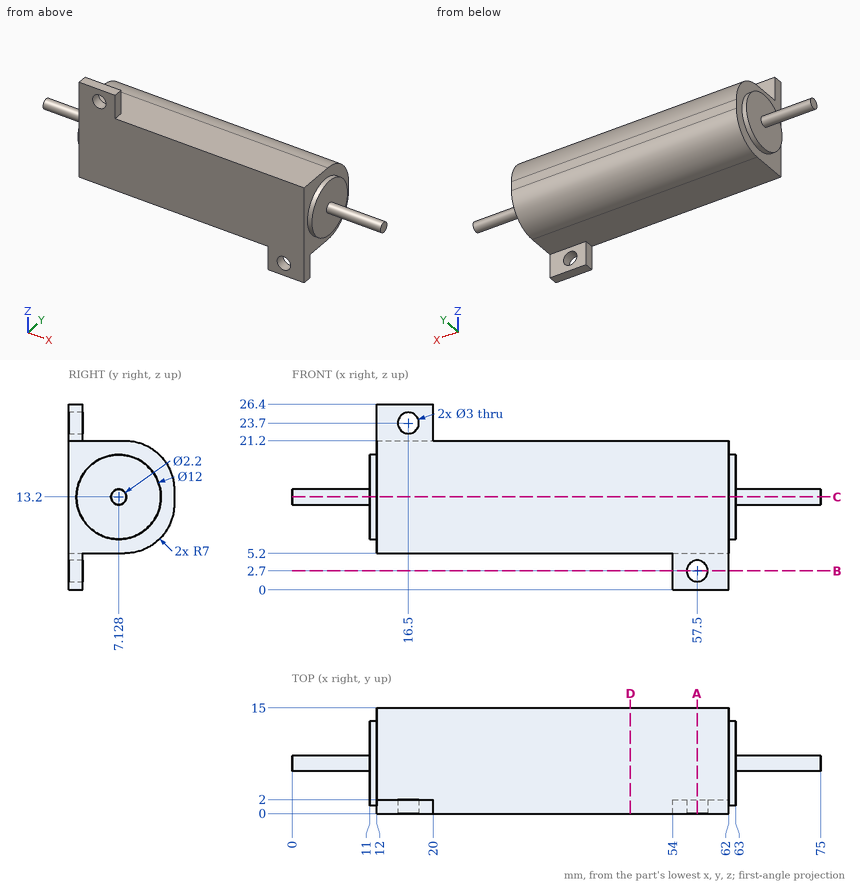
Design review of the part shown in the three views and the two pictorial views. Dimensions are in mm from the part's minimum x, y and z. Round coordinates to 2 decimals unless told otherwise and drop trailing zeros. Loops run counter-clockwise (first coordinate to the right, second up) from the corner with the lowest first, then second, coordinate; pieces in that order, holes last. Notation, with made-up numbers: M -18,57 L 40,57 A18 ccw 40,76 Z; hole C 74.5,49.5 d4. An arc over 180 degrees is marked long. Answer as a JSON object with one key per item and string values.
Item 1: Clearance check with flat-ended pins moving along their axes: P1, Ø1, axis at y = 1.5, z = 25, coming from the +X side; P2, Ø1.5, axis at x = 47.5, y = 12.5, coming from the +Z side; P3, Ø4, axis at y = 5.5, z = 6.5, coming from the +X side; P4, Ø3.5, axis at y = 9, z = 12, coming from the +X side. State where each tip first meets the part, or that it passes through.
Check sheet entries:
{"P1": "x = 20", "P2": "z = 20.11", "P3": "x = 63", "P4": "x = 75"}
Item 2: For line 1 along X through (y, z) = (0.5, 2.7); line 2 along X through (y, z) = (1.2, 23.7); line 3 along X through (y, z) = (0.5, 12.25), list the stretches that pass through material, from the lowest coordinate up.
Check sheet entries:
{"line 1": "54 to 56, 59 to 62", "line 2": "12 to 15, 18 to 20", "line 3": "12 to 62"}
Item 3: We need section D-D, the plane x = 48. State the section outline as (y, z) points.
Check sheet entries:
{"outline": "M 0,5.2 L 8,5.2 A7 ccw 15,12.2 L 15,14.2 A7 ccw 8,21.2 L 0,21.2 Z"}
Item 4: We need section B-B, the plane z = 2.7. State the section outline as (x, y) points.
Check sheet entries:
{"outline": "M 54,0 L 56,0 L 56,2 L 54,2 Z; M 59,0 L 62,0 L 62,2 L 59,2 Z"}
Item 5: We need section A-A, the plane x = 57.5. State the section outline as (y, z) points, and give its area (3 significant figures).
Check sheet entries:
{"outline": "M 0,0 L 2,0 L 2,1.2 L 0,1.2 Z; M 0,4.2 L 2,4.2 L 2,5.2 L 8,5.2 A7 ccw 15,12.2 L 15,14.2 A7 ccw 8,21.2 L 0,21.2 Z", "area": "223 mm2"}
Item 6: We need section C-C, the plane z = 13.2. State the section outline as (x, y) points, and give its area (3 significant figures).
Check sheet entries:
{"outline": "M 0,6.03 L 11,6.03 L 11,1.13 L 12,1.13 L 12,0 L 62,0 L 62,1.13 L 63,1.13 L 63,6.03 L 75,6.03 L 75,8.23 L 63,8.23 L 63,13.13 L 62,13.13 L 62,15 L 12,15 L 12,13.13 L 11,13.13 L 11,8.23 L 0,8.23 Z", "area": "825 mm2"}
